The model under review builds one solid part; all positions refer to its coordinate system, in mm. A direction names the side the tool comes from. Coordinates: 2 decimals unless noted, no trailing zeros. Order: outer loops, then holes, each group sorted by start corner. A loop starts at its lowest first (then second) coordinate and runs counter-clockwise, first axis right, second up. Notation, with made-up numbers: M 0.25,14.5 L 16.25,14.5 A16 ccw 16.25,39.5 Z; hole C 65.25,7.5 d3. An arc over 180 degrees is marked long. Write each question's results on one line, items separated by ' | '.
from build123d import *

# Parameters (mm, degrees)
F1_DEPTH = 10
F2_R     = 1
F3_W     = 6.485
F3_H     = 6.485
F4_DEPTH = 2.2


with BuildPart() as f1:
    # F0 (on Front) → F1 (new body)
    with BuildSketch(Plane.XZ):
        Polygon((-16.613121, 0), (-25.613121, 0), (0, -48.672046), (-0.281218, -19.773414), (-6.288659, -8.357607), (-5.897355, -20.351225), align=None)
    extrude(amount=F1_DEPTH)

    # F2
    f2_edges = [f1.edges().sort_by_distance(p)[0] for p in [
        (-12.806561, -10, -24.336023),
        (-11.255238, -10, -10.175613),
        (-6.093007, -10, -14.354416),
        (-3.284939, -10, -14.06551),
        (-0.140609, -10, -34.22273),
    ]]
    fillet(f2_edges, radius=F2_R)

    # F3 (on face) → F4 (join)
    with BuildSketch(Plane.XY):
        with Locations((-21.104121, -4.991)):
            Rectangle(F3_W, F3_H)
    extrude(amount=F4_DEPTH)


solid = f1.part
1) For faces 5 (the flat face through (-21, -8.234, 1)), 6 (the cylindrical face through (-0.43, -9.7, -34.02)), 7 (the flat face through (-21, -1.748, 1)), 8 (the flat face through (-17.862, -5, 1)), 9 (the flat face through (-21, -5, 2.2)), list the 3-axis set-ups (+Z, -Z, +X, -X, +Y, -Y) from which the entire face can be reached by the end or side of a thin tool; tool diameter is ignored.
Solutions:
face 5: +Z, +X, -X, -Y | face 6: +Z, +X, -Y | face 7: +Z, +X, -X, +Y | face 8: +Z, +X, +Y, -Y | face 9: +Z, +X, -X, +Y, -Y
2) For pin 1 (0.7 mm diameter, centred on x = -20, z = 1, fed in from +Y); pin 2 (1.8 mm diameter, centred on x = -22.5, z = 1, fed in from -Y); pin 3 (2 mm diameter, centred on x = -16.5, y = -3.5, fed in from +Z), all flat-tipped, find the tip position at first contact; note any pin that passes through.
Solutions:
pin 1: y = -1.75 | pin 2: y = -8.23 | pin 3: z = 0
3) To check wall thickness, follow line 1 along X through (y, z) = (-4, -13); line 2 along Y through (x, z) = (-17.75, -13); line 3 along X through (y, z) = (-6.5, -11). State the ranges of each line that lie inside material, in increasing order.
Solutions:
line 1: -18.77 to -9.77, -6.14 to -3.85 | line 2: -10 to 0 | line 3: -19.82 to -10.82, -6.2 to -4.9
4) Take a section at A-A on y = -5. State the section outline as (x, z) points, plus the area to 3 significant figures.
Solutions:
outline: M -25.61,0 L 0,-48.67 L -0.28,-19.77 L -6.29,-8.36 L -5.9,-20.35 L -16.61,0 L -17.86,0 L -17.86,2.2 L -24.35,2.2 L -24.35,0 Z | area: 440 mm2
5) Take a section at B-B on y = -1. State the section outline as (x, z) points, plus the area to 3 significant figures.
Solutions:
outline: M -25.61,0 L 0,-48.67 L -0.28,-19.77 L -6.29,-8.36 L -5.9,-20.35 L -16.61,0 Z | area: 426 mm2
6) The part is to be moulded in two halves that separate along X. For faces 1 (the flat face through (-24.347, -5, 1)), 2 (the cylindrical face through (-10.71, -9.7, -11.83)), 3 (the flat face through (-3.24, -4.44, -14.15)), 4 (the cylindrical face through (-5.73, -9.7, -16.63)), say which applies: pulls with the +X half, pulls with the -X half, needs draft (parallel to the pull), parting line crosses it, or undercut.
Solutions:
face 1: pulls with the -X half | face 2: undercut | face 3: pulls with the +X half | face 4: undercut
